Could you check a few things on this drawing? It's one solid part, dimensions in mm from its lowest x, y, z. A direction names the side the tool comes from. Give positions to 0.01 mm unless a question says otherwise; leave off trailing zeros. Order: outer loops, then holes, each group sorted by start corner. A loop starts at its lowest first (then second) coordinate and runs counter-clockwise, first axis right, second up.
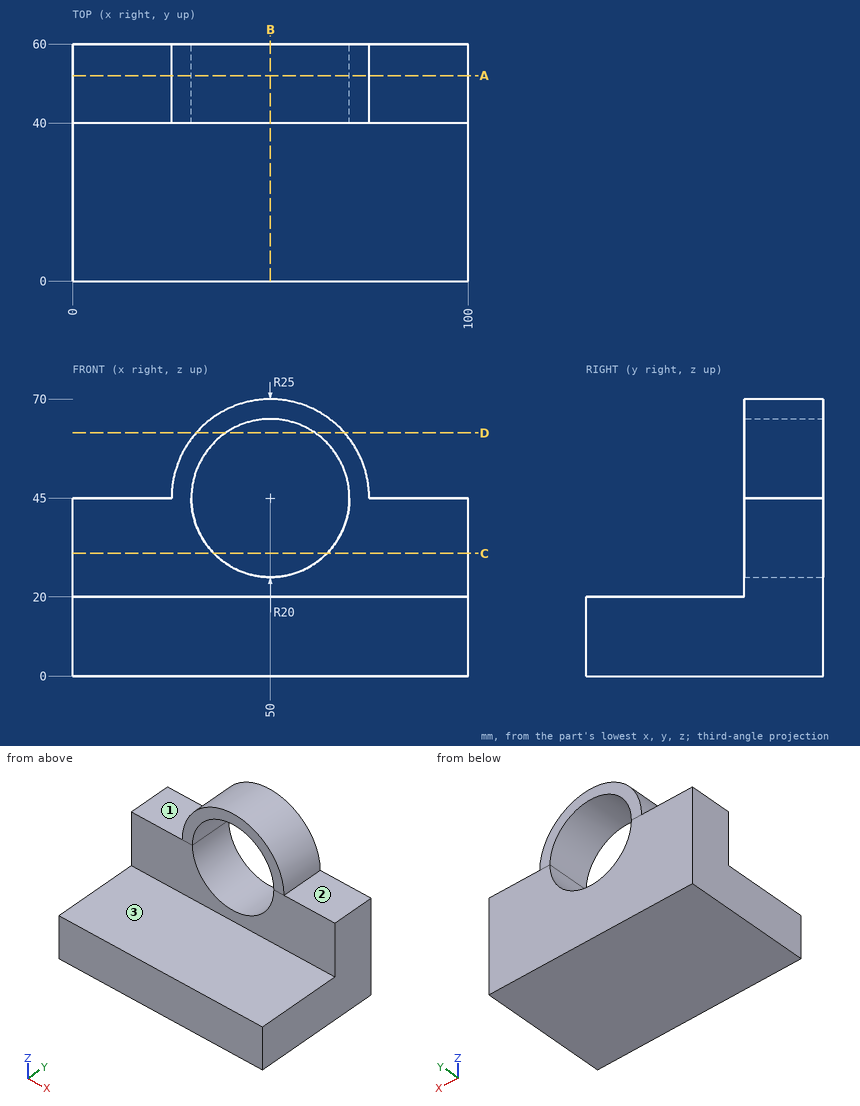
Item 1: Imagine slicing it at C-C on z = 31. List the corners of the cut face in (x, y) for me.
Findings:
outline: (0, 40) - (35.72, 40) - (35.72, 60) - (0, 60) - close; (64.28, 40) - (100, 40) - (100, 60) - (64.28, 60) - close
Item 2: Please list where these lines run through material, in increasing order: line 1 along Z through (x, y) = (14, 14.5); line 2 along Y through (x, z) = (7, 40); line 3 along Z through (x, y) = (84.5, 58).
Findings:
line 1: z = 0 to 20
line 2: y = 40 to 60
line 3: z = 0 to 45
Item 3: For the marked faces 1, 2 and 3, which set-ups out of +Z, -Z, +X, -X, +Y, -Y let a thin tool reach every point of the face, with its end or its side?
Findings:
face 1: +Z, -X, +Y, -Y
face 2: +Z, +X, +Y, -Y
face 3: +Z, +X, -X, -Y
Item 4: Imagine slicing it at B-B on x = 50. List the corners of the cut face in (y, z) for me, then the cut area to 3 significant figures.
Findings:
outline: (0, 0) - (60, 0) - (60, 25) - (40, 25) - (40, 20) - (0, 20) - close; (40, 65) - (60, 65) - (60, 70) - (40, 70) - close
area: 1,400 mm2
Item 5: Imagine slicing it at A-A on y = 52. List the corners of the cut face in (x, z) for me, then the cut area to 3 significant figures.
Findings:
outline: (0, 0) - (100, 0) - (100, 45) - (75, 45) arc R25 ccw to (25, 45) - (0, 45) - close; hole circle Ø40 at (50, 45)
area: 4,230 mm2
Item 6: Imagine slicing it at D-D on z = 61.5. List the corners of the cut face in (x, y) for me, then the cut area to 3 significant figures.
Findings:
outline: (31.22, 40) - (38.7, 40) - (38.7, 60) - (31.22, 60) - close; (61.3, 40) - (68.78, 40) - (68.78, 60) - (61.3, 60) - close
area: 299 mm2
Item 7: For pin 1 (6 mm diameter, centred on x = 74.5, z = 42, fed in from -Y); pin 2 (6 mm diameter, centred on x = 72, y = 8, fed in from +Z); pin 3 (16 mm diameter, centred on x = 15, y = 51, fed in from +Z), each with a flat end and sliding along its axis, tell me the tip position at first contact or that it passes through.
Findings:
pin 1: stops at y = 40
pin 2: stops at z = 20
pin 3: stops at z = 45
